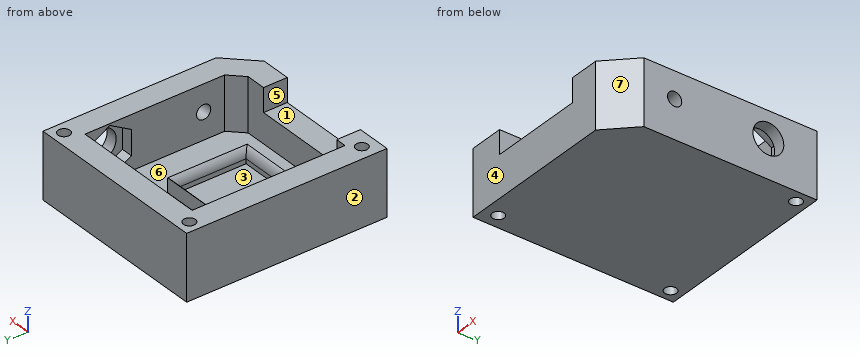
Autodesk Inventor part; units mm, degrees
ref_plane "YZ Plane" through (0, 0, 0) normal (1, 0, 0) x (0, 1, 0)
ref_plane "XZ Plane" through (0, 0, 0) normal (0, 1, 0) x (-1, 0, 0)
ref_plane "XY Plane" through (0, 0, 0) normal (0, 0, 1) x (1, 0, 0)
sketch "Sketch1" plane through (0, 0, 0) normal (0, 0, 1) x (1, 0, 0)
  line L0 (11.825, -16.125) -> (-11.825, -16.125)
  line L1 (-14.625, -13.325) -> (-14.625, 16.125)
  line L2 (-14.625, 16.125) -> (14.625, 16.125)
  line L3 (14.625, 16.125) -> (14.625, -13.325)
  line L4 (14.625, -16.125) -> (-14.625, 16.125) construction
  line L5 (-14.625, -16.125) -> (14.625, 16.125) construction
  line L6 (11.825, -16.125) -> (14.625, -13.325)
  line L7 (-14.625, -13.325) -> (-14.625, -16.125)
  line L8 (-11.825, -16.125) -> (-14.625, -16.125)
  point P0 (0, 0)
  dimension "d0" = 29.25
  dimension "d1" = 32.25
  dimension "d56" = 2.8
  dimension "d57" = 2.8
extrude "Extrusion1" add sketch "Sketch1" along normal blind 11.25
shell "Shell2" thickness 5 outward yes removed faces 1 at (-4.875, -3.5083, 11.25)
sketch "Sketch3" plane through (0, 0, 11.25) normal (0, 0, 1) x (1, 0, 0)
  line L0 (19.625, 21.125) -> (-19.625, 21.125) construction
  line L1 (-14.625, 16.125) -> (14.625, 16.125) construction
  line L2 (-19.625, 21.125) -> (-14.625, 16.125) construction
  line L3 (14.625, 16.125) -> (19.625, 21.125) construction
  line L4 (11.825, -16.125) -> (-14.625, -16.125) construction
  circle A0 centre (-17.125, 18.625) radius 1.25
  circle A1 centre (17.125, 18.625) radius 1.25
  line L5 (-14.625, -16.125) -> (-14.625, 16.125) construction
  line L6 (-14.625, -16.125) -> (-18.625, -20.125) construction
  circle A2 centre (-16.625, -18.125) radius 1.25
  point P0 (0, 0)
  point P1 (18.625, -20.125)
  point P2 (14.625, -16.125)
  point P3 (-11.825, -16.125)
  dimension "d14" = 2.5
  dimension "d15" = 2.5
  dimension "d58" = 2.5
extrude "Extrusion3" cut sketch "Sketch3" against normal through all
sketch "Sketch11" plane through (0, 0, 11.25) normal (0, 0, 1) x (1, 0, 0)
  line L0 (-19.625, -21.125) -> (13.8961, -21.125)
  line L1 (-14.625, -16.125) -> (11.825, -16.125)
  line L2 (7.625, -21.125) -> (-12.375, -21.125)
  line L3 (-12.375, -21.125) -> (-12.375, -16.125)
  line L4 (-12.375, -16.125) -> (7.625, -16.125)
  line L5 (7.625, -16.125) -> (7.625, -21.125)
  circle A0 centre (-16.625, -18.125) radius 1.25
  line L6 (-19.625, 21.125) -> (-19.625, -21.125)
  point P0 (0, 0)
  point P1 (-13.4819, -20.125)
  point P2 (18.625, -20.125)
  point P3 (-11.825, -16.125)
  point P4 (14.625, -16.125)
  point P5 (13.8961, -21.125)
  point P6 (7.625, -16.125)
  dimension "d60" = 20
  dimension "d87" = 7.25
extrude "Extrusion11" cut sketch "Sketch11" against normal blind 5 contours L3 L1 L5 L0
sketch "Sketch13" plane through (19.625, -15.3961, -5) normal (1, 0, 0) x (0, 0, -1)
  line L0 (-11.5, 18.8569) -> (-11.5, 3.8569) construction
  circle A0 centre (-10.625, 26.2711) radius 3.25
  line L1 (-16.25, 0) -> (-16.25, 36.5211) construction
  line L2 (0, 0) -> (-16.25, 0) construction
  line L3 (0, 36.5211) -> (-16.25, 36.5211)
  line L4 (-5, 2.0711) -> (-5, 31.5211)
  point P0 (-5, 15.3961)
  dimension "d61" = 6.5
  dimension "d81" = 10.25
  dimension "d86" = 5.625
extrude "Extrusion13" cut sketch "Sketch13" against normal up to surface (5 mm away)
sketch "Sketch14" plane through (-14.625, 16.125, 0) normal (0, 0, 1) x (1, 0, 0)
  line L0 (2, -11.5) -> (19.25, -11.5)
  line L1 (19.25, -11.5) -> (19.25, -26.25)
  line L2 (19.25, -26.25) -> (2, -26.25)
  line L3 (2, -26.25) -> (2, -11.5)
  line L4 (1.25, -10.5) -> (20, -10.5)
  line L5 (20.25, -11.25) -> (20.25, -27)
  line L6 (19.45, -27.25) -> (1.25, -27.25)
  line L7 (1, -27) -> (1, -10.75)
  line L8 (0, -32.25) -> (0, 0)
  line L9 (2.25, -32.25) -> (0, -32.25)
  line L10 (20, -10.5) -> (20.25, -10.5)
  line L11 (20.25, -10.5) -> (20.25, -11.25)
  line L12 (19.45, -27.25) -> (20.25, -27.25)
  line L13 (20.25, -27.25) -> (20.25, -27)
  line L14 (1.25, -27.25) -> (1, -27.25)
  line L15 (1, -27) -> (1, -27.25)
  line L16 (1, -10.75) -> (1, -10.5)
  line L17 (1.25, -10.5) -> (1, -10.5)
  point P0 (14.625, -16.125)
  point P1 (10.625, -11.5)
  point P2 (10.625, -10.5)
  point P3 (1, -18.875)
  point P4 (2, -18.875)
  dimension "d66" = 1
  dimension "d67" = 1
  dimension "d69" = 17.25
  dimension "d70" = 14.75
  dimension "d71" = 1
  dimension "d72" = 5
  dimension "d83" = 1
  dimension "d84" = 1
extrude "Extrusion14" add sketch "Sketch14" along normal blind 3
sketch "Sketch15" plane through (0, 0, -5) normal (0, 0, -1) x (-1, 0, 0)
  line L0 (-19.625, -15.3961) -> (-19.625, 21.125)
  line L1 (19.625, -21.125) -> (-13.8961, -21.125)
  line L2 (-19.625, 21.125) -> (19.625, 21.125)
  line L3 (19.625, 21.125) -> (19.625, -21.125)
  line L4 (19.625, -21.125) -> (-19.625, -21.125)
  line L5 (-19.625, -21.125) -> (-19.625, 21.125)
  point P0 (0, 0)
extrude "Extrusion15" cut sketch "Sketch15" against normal blind 2.5
sketch "Sketch16" plane through (19.625, -15.3961, 11.25) normal (1, 0, 0) x (0, 0, -1)
  point P0 (11.25, 15.3961)
sketch "Sketch17" plane through (19.625, -15.3961, 11.25) normal (1, 0, 0) x (0, 0, -1)
  circle A0 centre (5.625, 6.5) radius 1.5
  circle A1 centre (5.625, 26.2711) radius 3.25
  line L0 (13.75, 0) -> (0, 0)
  point P0 (11.25, 15.3961)
  point P1 (0.8377, 31.1069)
  point P2 (7.1623, 31.1069)
  dimension "d77" = 3
  dimension "d82" = 6.5
extrude "Extrusion16" cut sketch "Sketch17" against normal up to surface (5 mm away) contours A0
fillet "Fillet1" radius 2.5 4 edges at (-4, 4.625, 3) (-12.625, -2.75, 3) (-4, -10.125, 3) (4.625, -2.75, 3)
sketch "Sketch18" plane through (14.625, -13.325, 0) normal (-1, 0, 0) x (0, 0, 1)
  circle A0 centre (5.625, 24.2) radius 3.25 construction
  circle A1 centre (5.625, 24.2) radius 4.55 construction
  line L0 (7.0809, 28.75) -> (11.4566, 28.75) construction
  line L1 (5.625, 28.75) -> (5.625, 19.65) construction
  line L2 (1.075, 24.2) -> (10.175, 24.2) construction
  line L3 (5.625, 24.2) -> (10.175, 24.2) construction
  line L4 (10.175, 24.2) -> (11.25, 24.2) construction
  line L5 (11.25, 29.45) -> (11.25, 0) construction
  line L6 (8.2519, 28.75) -> (10.8789, 24.2)
  line L7 (10.8789, 24.2) -> (8.2519, 19.65)
  line L8 (8.2519, 19.65) -> (2.9981, 19.65)
  line L9 (2.9981, 19.65) -> (0.3711, 24.2)
  line L10 (0.3711, 24.2) -> (2.9981, 28.75)
  line L11 (2.9981, 28.75) -> (8.2519, 28.75)
  point P0 (0, 13.325)
  point P1 (9.0965, 27.1413)
  dimension "d88" = 9.1
extrude "Extrusion17" cut sketch "Sketch18" against normal blind 2.5
equation "\"d57\" = d56"
equation "\"d58\" = d14"
equation "\"d86\" = 0.5 * d4"
equation "\"d71\" = d67"
equation "\"d83\" = d67"
equation "\"d84\" = d67"
equation "\"d92\" = 0.5 * d13"
properties part number "AmpClipOn"
Geometry check sheet. Reference: the model listing, model coordinates, mm. Face numbers are marked on the shaded views. A direction names the side the tool comes from. Round coordinates to 2 decimals unless told otherwise and drop trailing zeros. Order: outer loops, then holes, each group sorted by start corner. A loop starts at its lowest first (then second) coordinate and runs counter-clockwise, first axis right, second up. Notation, with made-up numbers: (-2, 38) -> (55, 38) arc R24 cw to (55, 57) -> close; hole circle Ø7 at (69.25, 32). An arc over 180 degrees is marked (long way). Return JSON: item names as keys, results as strings. Group by question number.
Q1. Tool access check on the marked faces 1, 2 and 3. Record the directions out of +Z, -Z, +X, -X, +Y, -Y that give a thin tool (end or side, any length) a straight path to the whole face; none if there is none.
Q2. Section check B-B, the plane y = -1. Record the boundary of the cut face in (x, z) (3 decimals).
Q3. Gauge pin test, flat ends, axial feed: pin 1 (3 mm diameter, centred on y = 11, z = 5, fed in from +X) (3 decimals); pin 2 (5.5 mm diameter, centred on x = -3.5, y = -20, fed in from +Z); pin 3 (2 mm diameter, centred on x = 16.5, z = 5, fed in from -Y). Record the tip position at first contact, or that the pin passes through.
Q4. Section check D-D, the plane x = 9. Record the boundary of the cut face in (y, z) (3 decimals).
Q5. Release check for a two-part mould opening along X. For the marked faces 4, 5, 6 and 7 record: released by +X, released by -X, zero draft, split by the parting line, or undercut.
Q6. Material ranges on probe 1 along Y at (x, z) = (-0.5, 5) (3 decimals); probe 2 along Y at (x, z) = (-5, 1) (3 decimals); probe 3 along Y at (x, z) = (-7.5, 1.75) (3 decimals), recorded low to high. Write a range as from..to.
Q7. Section check C-C, the plane x = -17. Record the boundary of the cut face in (y, z) (3 decimals).
Q8. Section check A-A, the plane x = -1. Record the boundary of the cut face in (y, z) (3 decimals).
Numbers:
{
 "1": {"face 1": "+Z, -Y", "face 2": "+Z, -Z, -X, +Y, -Y", "face 3": "+Z"},
 "2": {"outline": "(-19.625, -2.5) -> (19.625, -2.5) -> (19.625, 11.25) -> (14.625, 11.25) -> (14.625, 0) -> (5.625, 0) -> (5.625, 3) arc R2.5 ccw to (4.625, 1) -> (4.625, 0) -> (-12.625, 0) -> (-12.625, 1) arc R2.5 ccw to (-13.625, 3) -> (-13.625, 0) -> (-14.625, 0) -> (-14.625, 11.25) -> (-19.625, 11.25) -> close"},
 "3": {"pin 1": "x = -14.625", "pin 2": "z = 6.25", "pin 3": "y = -19.52"},
 "4": {"outline": "(-21.125, -2.5) -> (21.125, -2.5) -> (21.125, 11.25) -> (16.125, 11.25) -> (16.125, 0) -> (-16.125, 0) -> (-16.125, 11.25) -> (-21.125, 11.25) -> close"},
 "5": {"face 4": "zero draft", "face 5": "undercut", "face 6": "undercut", "face 7": "released by +X"},
 "6": {"probe 1": "-21.125..-16.125, 16.125..21.125", "probe 2": "-21.125..-16.125, -11.125..-10.125, 4.625..5.625, 16.125..21.125", "probe 3": "-21.125..-16.125, -11.125..-10.24, 4.74..5.625, 16.125..21.125"},
 "7": {"outline": "(-21.125, -2.5) -> (-19.317, -2.5) -> (-19.317, 11.25) -> (-21.125, 11.25) -> close; (-16.933, -2.5) -> (17.381, -2.5) -> (17.381, 11.25) -> (-16.933, 11.25) -> close; (19.869, -2.5) -> (21.125, -2.5) -> (21.125, 11.25) -> (19.869, 11.25) -> close"},
 "8": {"outline": "(-21.125, -2.5) -> (21.125, -2.5) -> (21.125, 11.25) -> (16.125, 11.25) -> (16.125, 0) -> (5.625, 0) -> (5.625, 3) arc R2.5 ccw to (4.625, 1) -> (4.625, 0) -> (-10.125, 0) -> (-10.125, 1) arc R2.5 ccw to (-11.125, 3) -> (-11.125, 0) -> (-16.125, 0) -> (-16.125, 6.25) -> (-21.125, 6.25) -> close"}
}
